Work out the finished part from the listing and answer in its coordinate system (mm). A direction names the side the tool comes from. Give positions to 0.01 mm unless a question says otherwise; leave off trailing zeros. Order: outer loops, then holes, each group sorted by start corner. A loop starts at its lowest first (then second) coordinate and runs counter-clockwise, first axis right, second up. Notation, with made-up numbers: (56.5, 3.5) - (102.5, 3.5) arc R20 ccw to (102.5, 30.5) - close; hole circle Ø10 at (10.5, 59). An arc over 180 degrees is marked (long way). Put each result on its own line as item: value.
```python
from build123d import *

# Parameters (mm, degrees)
EXTRUDE_THIN1_DEPTH            = 510
EXTRUDE_THIN1_DEPTH_BACK       = 280
SKETCH1_W                      = 76.2
SKETCH1_H                      = 38.1
SKETCH1_W_2                    = 69.85
SKETCH1_H_2                    = 31.75
CUT_EXTRUDE1_REACH             = 514.838
SKETCH6_R                      = 22.225
F_12_0_12_DIAMETER_HOLE2_D     = 12
F_12_0_12_DIAMETER_HOLE2_DEPTH = 3.175
F_12_0_12_DIAMETER_HOLE1_D     = 12
F_12_0_12_DIAMETER_HOLE1_DEPTH = 3.175
CUT_EXTRUDE2_REACH             = 514.838
SKETCH7_R                      = 22.225


with BuildPart() as part:
    # Sketch1 → Extrude-Thin1 (new, two sides: drawn at the far end of the back side and taken through both)
    with BuildSketch(Plane(origin=(0, 0, 0), x_dir=(1, 0, 0), z_dir=(0, 1, 0)).offset(-EXTRUDE_THIN1_DEPTH_BACK)):
        Rectangle(SKETCH1_W, SKETCH1_H)
        Rectangle(SKETCH1_W_2, SKETCH1_H_2, mode=Mode.SUBTRACT)
    extrude(amount=EXTRUDE_THIN1_DEPTH + EXTRUDE_THIN1_DEPTH_BACK)

    # Sketch6 → Cut-Extrude1 (cut, up to next)
    with BuildSketch(Plane.XY.offset(19.05), mode=Mode.PRIVATE) as cut_extrude1_sk1:
        with Locations((6.511806663, 446.930290738)):
            Circle(SKETCH6_R)
    cut_extrude1_tool1 = extrude(cut_extrude1_sk1.sketch, amount=-CUT_EXTRUDE1_REACH, mode=Mode.PRIVATE) & part.part
    # Sketch6 → Cut-Extrude1 (cut, up to next)
    with BuildSketch(Plane.XY.offset(19.05), mode=Mode.PRIVATE) as cut_extrude1_sk2:
        with Locations((-6.511806663, 373.069709262)):
            Circle(SKETCH6_R)
    cut_extrude1_tool2 = extrude(cut_extrude1_sk2.sketch, amount=-CUT_EXTRUDE1_REACH, mode=Mode.PRIVATE) & part.part
    add(cut_extrude1_tool1.solids().sort_by_distance((6.511807, 446.930291, 19.05))[0], mode=Mode.SUBTRACT)
    add(cut_extrude1_tool2.solids().sort_by_distance((-6.511807, 373.069709, 19.05))[0], mode=Mode.SUBTRACT)

    # Ø12.0 (12) Diameter Hole2
    with Locations(Plane.XY.offset(19.05)):
        with Locations((-20, 485), (20, 485), (-20, 335)):
            Hole(F_12_0_12_DIAMETER_HOLE2_D / 2, depth=F_12_0_12_DIAMETER_HOLE2_DEPTH)

    # Ø12.0 (12) Diameter Hole1
    with Locations(Plane(origin=(0, 0, -19.05), x_dir=(-1, 0, 0), z_dir=(0, 0, -1))):
        with Locations((-20, -15), (20, -255), (-20, -255), (20, -15)):
            Hole(F_12_0_12_DIAMETER_HOLE1_D / 2, depth=F_12_0_12_DIAMETER_HOLE1_DEPTH)

    # Sketch7 → Cut-Extrude2 (cut, up to next)
    with BuildSketch(Plane(origin=(0, 0, -19.05), x_dir=(-1, 0, 0), z_dir=(0, 0, -1)), mode=Mode.PRIVATE) as cut_extrude2_sk1:
        with Locations((0, -50)):
            Circle(SKETCH7_R)
    cut_extrude2_tool1 = extrude(cut_extrude2_sk1.sketch, amount=-CUT_EXTRUDE2_REACH, mode=Mode.PRIVATE) & part.part
    # Sketch7 → Cut-Extrude2 (cut, up to next)
    with BuildSketch(Plane(origin=(0, 0, -19.05), x_dir=(-1, 0, 0), z_dir=(0, 0, -1)), mode=Mode.PRIVATE) as cut_extrude2_sk2:
        with Locations((0, -220)):
            Circle(SKETCH7_R)
    cut_extrude2_tool2 = extrude(cut_extrude2_sk2.sketch, amount=-CUT_EXTRUDE2_REACH, mode=Mode.PRIVATE) & part.part
    add(cut_extrude2_tool1.solids().sort_by_distance((0, -50, -19.05))[0], mode=Mode.SUBTRACT)
    add(cut_extrude2_tool2.solids().sort_by_distance((0, -220, -19.05))[0], mode=Mode.SUBTRACT)


solid = part.part
```
(1) A tool of negligible diameter and unlimited length cuts with its end or side. For faces 1 (the face through (-1, 109, 19.05)), 2 (the face through (-34.925, 109, 0)), 3 (the face through (-19.22, 490.95, 17.44)), 4 (the face through (4.8, -241.7, -17.5)), from which of +Z, -Z, +X, -X, +Y, -Y can it reach the whole face along a straight path? Write none if from no direction.
Geometry check:
face 1: +Z, +X, -X, +Y, -Y
face 2: +Y, -Y
face 3: +Z
face 4: -Z
(2) Straight lines are drawn through the part: line 1 (Y direction, x = 0, z = -16.7) (3 decimals); line 2 (X direction, y = 485, z = 16); line 3 (X direction, y = 359, z = 7.5) (3 decimals). For each, find the intervals that lie inside material, in ascending order.
Geometry check:
line 1: y = -280 to -242.225, -197.775 to -72.225, -27.775 to 510
line 2: x = -38.1 to -26, -14 to 14, 26 to 38.1
line 3: x = -38.1 to -34.925, 34.925 to 38.1
(3) Section B-B, the plane y = -113.5 is taken. Write down the section's boundary in (x, z) (3 decimals), then the cut area to 3 significant figures.
Geometry check:
outline: (-38.1, -19.05) - (38.1, -19.05) - (38.1, 19.05) - (-38.1, 19.05) - close; hole (-34.925, -15.875) - (34.925, -15.875) - (34.925, 15.875) - (-34.925, 15.875) - close
area: 685 mm²
(4) Section A-A, the plane z = -9 is taken. Write down the section's boundary in (x, y) (3 decimals), then the cut area to 3 significant figures.
Geometry check:
outline: (-38.1, -280) - (-34.925, -280) - (-34.925, 510) - (-38.1, 510) - close; (34.925, -280) - (38.1, -280) - (38.1, 510) - (34.925, 510) - close
area: 5,020 mm²
(5) Given pin 1 (7 mm diameter, centred on x = -20, y = -15, fed in from -Z) (3 decimals), flat-ended and moving along its own axis, determine where the tip first touches the part or whether it passes through.
Geometry check:
pin 1: stops at z = 15.875
(6) Section D-D, the plane y = -220 is taken. Write down the section's boundary in (x, z) (3 decimals), then the cut area to 3 significant figures.
Geometry check:
outline: (-38.1, -19.05) - (-22.225, -19.05) - (-22.225, -15.875) - (-34.925, -15.875) - (-34.925, 15.875) - (34.925, 15.875) - (34.925, -15.875) - (22.225, -15.875) - (22.225, -19.05) - (38.1, -19.05) - (38.1, 19.05) - (-38.1, 19.05) - close
area: 544 mm²
(7) Section C-C, the plane x = 1 is taken. Count the separate pieces of the cut face and the enclosed holes in it, then the cut area to 3 significant figures.
Geometry check:
separate pieces: 6
enclosed holes: 0
area: 4,460 mm²
(8) Determine the mould class of faces 5 (the face through (23.226, -9.941, -17.44)), 6 (the face through (0, 109, -15.875)), 7 (the face through (-3, -280, 17)), 8 (the face through (-24.42, -10.94, -17.44)) for opening direction Y: pulls with the +Y half, pulls with the -Y half, needs draft (parallel to the pull), parting line crosses it, or undercut.
Geometry check:
face 5: undercut
face 6: needs draft
face 7: pulls with the -Y half
face 8: undercut
